```python
from build123d import *

# Parameters (mm, degrees)
F1_DEPTH = 210
F3_D     = 9
F3_DEPTH = 12
F3_TIP   = 2.7038727856
F5_DEPTH = 95
F7_D     = 9
F7_DEPTH = 12
F7_TIP   = 2.7038727856
F9_D     = 10.5
F9_DEPTH = 12
F9_TIP   = 3.1545182499


with BuildPart() as f1:
    # F0 (on Right) → F1 (new body)
    with BuildSketch(Plane.YZ):
        with BuildLine():
            Line((-3, 0), (0, 0))
            Line((0, 0), (0, 30))
            Line((0, 30), (-30, 30))
            Line((-30, 30), (-30, 27))
            Line((-30, 27), (-6, 27))
            ThreePointArc((-6, 27), (-3.8786796564, 26.1213203436), (-3, 24))
            Line((-3, 24), (-3, 0))
        make_face()
    extrude(amount=F1_DEPTH)

    # F3
    with Locations(Plane.XZ.offset(3)):
        with Locations((36, 12), (174, 12)):
            Hole(F3_D / 2, depth=F3_DEPTH)
            with Locations((0, 0, -(F3_DEPTH + F3_TIP / 2))):  # 118° drill point
                Cone(0, F3_D / 2, F3_TIP, mode=Mode.SUBTRACT)

    # F4 (on face) → F5 (cut)
    with BuildSketch(Plane.XZ.offset(30)):
        Polygon((30, 0), (3, 27), (0, 27), (0, 0), align=None)
        Polygon((3, 27), (0, 30), (0, 27), align=None)
        Polygon((210, 27), (210, 30), (207, 27), align=None)
        Polygon((210, 27), (207, 27), (180, 0), (210, 0), align=None)
    extrude(amount=-F5_DEPTH, mode=Mode.SUBTRACT)

    # F7
    with Locations(Plane(origin=(0, 0, 27), x_dir=(1, 0, 0), z_dir=(0, 0, -1))):
        with Locations((15, 15), (195, 15)):
            Hole(F7_D / 2, depth=F7_DEPTH)
            with Locations((0, 0, -(F7_DEPTH + F7_TIP / 2))):  # 118° drill point
                Cone(0, F7_D / 2, F7_TIP, mode=Mode.SUBTRACT)

    # F9
    with Locations(Plane(origin=(0, 0, 27), x_dir=(1, 0, 0), z_dir=(0, 0, -1))):
        with Locations((172, 15)):
            Hole(F9_D / 2, depth=F9_DEPTH)
            with Locations((0, 0, -(F9_DEPTH + F9_TIP / 2))):  # 118° drill point
                Cone(0, F9_D / 2, F9_TIP, mode=Mode.SUBTRACT)


solid = f1.part
```
Geometry check sheet. Reference: the model listing, model coordinates, mm. A direction names the side the tool comes from. Give positions to 0.01 mm unless a question says otherwise; leave off trailing zeros. Order: outer loops, then holes, each group sorted by start corner. A loop starts at its lowest first (then second) coordinate and runs counter-clockwise, first axis right, second up. Notation, with made-up numbers: (23, 61.5) - (60, 61.5) arc R18 cw to (60, 70.5) - close; hole circle Ø11 at (84, -12.75). An arc over 180 degrees is marked (long way). Write item = value, one per line. Start each with the question number.
1) Section check A-A (x = 195). Enter the section's corners in (y, z), then the cut area to 3 significant figures.
2) Section check B-B (z = 12). Enter the section's corners in (x, y), then the cut area to 3 significant figures.
3) Access from +Z, -Z, +X, -X, +Y, -Y to the whole of each face (thin tool, end or side, straight path). Record for faces 1 (the flat face through (201.7, -2.8, 21.7)), 2 (the flat face through (104, -18, 27)).
4) Draft check along Z on faces 3 (the flat face through (104, -15, 30)), 4 (the flat face through (104, -3, 12)), 5 (the cylindrical face through (169.84, -1.48, 10.28)). Enter one of: released by +Z, released by -Z, zero draft, split by the parting line, or undercut.
5) Gauge pin test, flat ends, axial feed: pin 1 Ø6 at (x, z) = (132, 8.5) entering from +Y; pin 2 Ø5 at (x, z) = (149.5, 5.5) entering from -Y; pin 3 Ø7 at (x, y) = (84, -13.5) entering from -Z. Record the tip position at first contact, or that the pin passes through.
6) Section check C-C (x = 28). Enter the section's corners in (y, z).
7) Section check D-D (y = -25). Enter the section's corners in (x, z), then the cut area to 3 significant figures.
8) Scan lines: L1, parallel to Z at x = 174, y = -1; L2, parallel to Y at x = 172, z = 28.25; L3, parallel to Z at x = 23.5, y = -8.5. Record each from-to range of solid material in increasing order.
Geometry check:
q1.outline = (-30, 27) - (-19.5, 27) - (-19.5, 30) - (-30, 30) - close; (-10.5, 27) - (-6, 27) arc R3 cw to (-3, 24) - (-3, 15) - (0, 15) - (0, 30) - (-10.5, 30) - close
q1.area = 101 mm2
q2.outline = (18, -3) - (31.5, -3) - (31.5, 0) - (18, 0) - close; (40.5, -3) - (169.5, -3) - (169.5, 0) - (40.5, 0) - close; (178.5, -3) - (192, -3) - (192, 0) - (178.5, 0) - close
q2.area = 468 mm2
q3.face_1 = -Z, +X, +Y, -Y
q3.face_2 = -Z, +X, -X, -Y
q4.face_3 = released by +Z
q4.face_4 = zero draft
q4.face_5 = undercut
q5.pin_1 = 0
q5.pin_2 = -3
q5.pin_3 = 27
q6.outline = (-30, 27) - (-6, 27) arc R3 cw to (-3, 24) - (-3, 2) - (0, 2) - (0, 30) - (-30, 30) - close
q7.outline = (0, 30) - (3, 27) - (207, 27) - (210, 30) - close
q7.area = 621 mm2
q8.L1 = 0 to 7.5, 16.5 to 30
q8.L2 = -30 to -20.25, -9.75 to 0
q8.L3 = 27 to 30
